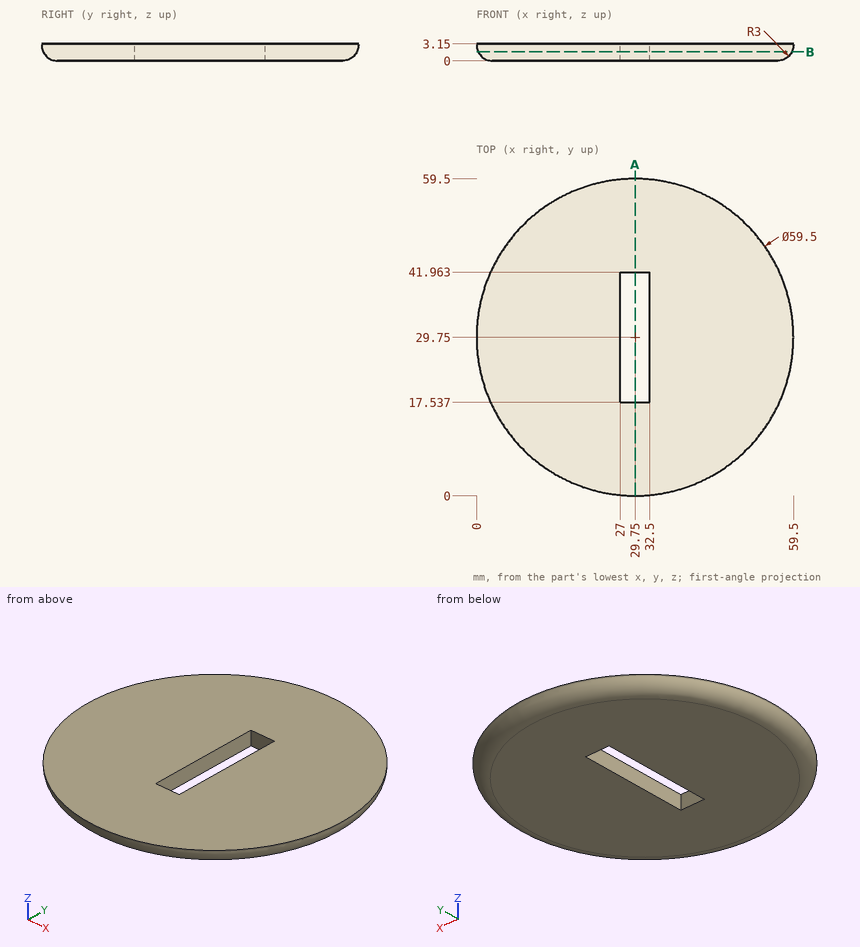
Drawing for the job (mm, zero at the part's lowest x, y, z). Give positions to 0.01 mm unless a question says otherwise; leave off trailing zeros. Loops run counter-clockwise (first coordinate to the right, second up) from the corner with the lowest first, then second, coordinate; pieces in that order, holes last.
Item 1: Slice it at A-A (x = 29.75). Write the cut outline in (y, z), plus the area to 3 significant figures.
Check values:
outline: (0, 3) arc R3 ccw to (3, 0) - (17.54, 0) - (17.54, 3.15) - (0, 3.15) - close; (41.96, 0) - (56.5, 0) arc R3 ccw to (59.5, 3) - (59.5, 3.15) - (41.96, 3.15) - close
area: 107 mm2
Item 2: Drill centre lines: line 1 along X through (y, z) = (22, 1.05); line 2 along X through (y, z) = (41, 2.7) (1 decimal); line 3 along Y through (x, z) = (32, 0.7). Where is each one in solid material? Low to high.
Check values:
line 1: x = 1.77 to 27, 32.5 to 57.73
line 2: x = 2.2 to 27, 32.5 to 57.3
line 3: y = 1.16 to 17.54, 41.96 to 58.34
Item 3: Drop flat-ended pins along their axis: P1, Ø0.9, axis at y = 31, z = 2, coming from the -X side (1 decimal); P2, Ø1.5, axis at x = 34.5, z = 2.5, coming from the +Y side; P3, Ø1.5, axis at y = 22.5, z = 2.5, coming from the -X side. Give the stop position or say it passes through.
Check values:
P1: stops at x = 0.1
P2: stops at y = 59.21
P3: stops at x = 0.74
Item 4: Slice it at B-B (z = 1.65). Write the cut outline in (x, y), plus the area to 3 significant figures.
Check values:
outline: circle Ø58.86 at (29.75, 29.75); hole (27, 17.54) - (32.5, 17.54) - (32.5, 41.96) - (27, 41.96) - close
area: 2,590 mm2
